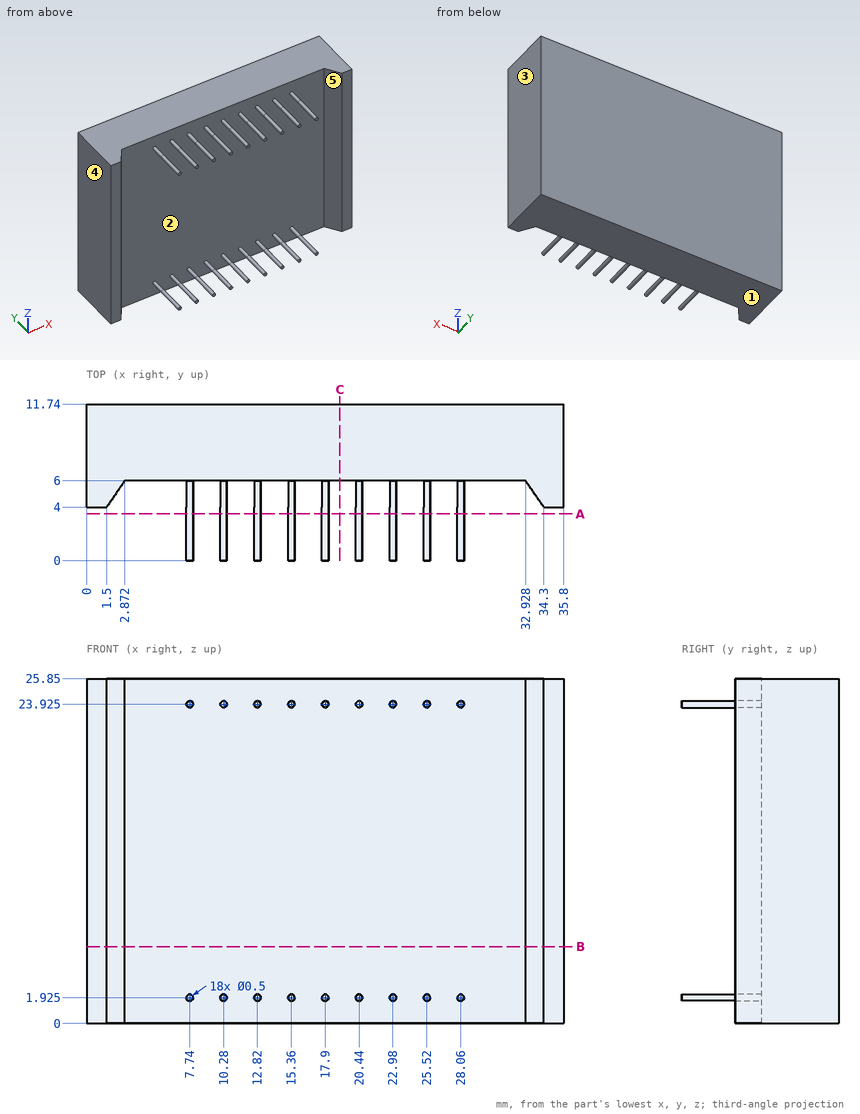
Could you check a few things on this drawing? It's one solid part, dimensions in mm from its lowest x, y, z. A direction names the side the tool comes from. Give positions to 0.01 mm unless a question says otherwise; leave off trailing zeros. Write each loop counter-clockwise with the first axis right and the second up, starting at its lowest first coordinate (ties: lowest second). Pieces come first, ordered by that corner, then holes. Notation, with made-up numbers: (-20.75, 23) -> (18.25, 23) arc R25 ccw to (18.25, 38) -> close; hole circle Ø5 at (21.5, 50). An arc over 180 degrees is marked (long way). Write each question's results on one line, items separated by ' | '.
1. I want a section at A-A, the plane y = 3.5. Count the separate pieces of the cut face and the enclosed holes in it.
Check sheet entries:
separate pieces: 18 | enclosed holes: 0
2. If we mould it in two halves opening along X, with no side actions, what happens to the marked faces 1, 2 and 3? For each: released by +X, released by -X, zero draft, split by the parting line, or undercut.
Check sheet entries:
face 1: zero draft | face 2: undercut | face 3: released by +X
3. I want a section at C-C, the plane x = 19. Write out the boundary of the cut face in (y, z).
Check sheet entries:
outline: (6, 0) -> (11.74, 0) -> (11.74, 25.85) -> (6, 25.85) -> close
4. On a 3-axis mill with a long thin cutter (end or side, diameter ignored), from which of +Z, -Z, +X, -X, +Y, -Y can I reach the whole of each face in a straight line? I mean the marked faces 4 and 5. Say none if no direction works.
Check sheet entries:
face 4: +Z, -Z, -X, +Y, -Y | face 5: +Z, -Z, -Y
5. Will these pins go through, and if not, where does the flat tip stop? pin 1 Ø0.8 at (x, z) = (0.5, 13) entering from -Y; pin 2 Ø3 at (x, z) = (25.5, 21.5) entering from -Y.
Check sheet entries:
pin 1: stops at y = 4 | pin 2: stops at y = 6
6. I need wall thicknesses on L1, parallel to Z at x = 20.5, y = 1.5; L2, parallel to Y at x = 23, z = 22; L3, parallel to X at y = 4.5, z = 22.25. Which ranges of each line are inside material? Lowest first, please.
Check sheet entries:
L1: z = 1.68 to 2.17, 23.68 to 24.17 | L2: y = 6 to 11.74 | L3: x = 0 to 1.84, 33.96 to 35.8
7. I want a section at B-B, the plane z = 5.75. Write out the boundary of the cut face in (x, y), then the cut area to 3 significant figures.
Check sheet entries:
outline: (0, 4) -> (1.5, 4) -> (2.87, 6) -> (32.93, 6) -> (34.3, 4) -> (35.8, 4) -> (35.8, 11.74) -> (0, 11.74) -> close | area: 214 mm²
